```python
from build123d import *

# Parameters (mm, degrees)
SKETCH1_W           = 152.4
SKETCH1_H           = 76.2
BOSS_EXTRUDE1_DEPTH = 25.4
SKETCH2_R           = 6.35
CUT_EXTRUDE1_DEPTH  = 89.9
SKETCH3_R           = 28.575
BOSS_EXTRUDE2_DEPTH = 19.05
SKETCH4_R           = 15.875
CUT_EXTRUDE3_DEPTH  = 97.092936785
FILLET1_R           = 6.35
CHAMFER1_SIZE       = 3.175


with BuildPart() as part:
    # Sketch1 → Boss-Extrude1 (new body)
    with BuildSketch(Plane(origin=(0, 0, 0), x_dir=(1, 0, 0), z_dir=(0, 1, 0))):
        Rectangle(SKETCH1_W, SKETCH1_H)
    extrude(amount=BOSS_EXTRUDE1_DEPTH)

    # Sketch2 → Cut-Extrude1 (cut, through all)
    with BuildSketch(Plane(origin=(0, 25.4, 0), x_dir=(1, 0, 0), z_dir=(0, 1, 0))):
        with Locations(Location((-57.15, 19.05, 0), (0, 0, 270))):
            Circle(SKETCH2_R)
        with Locations(Location((-57.15, -19.05, 0), (0, 0, 90))):
            Circle(SKETCH2_R)
        with Locations(Location((57.15, -19.05, 0), (0, 0, 270))):
            Circle(SKETCH2_R)
        with Locations(Location((57.15, 19.05, 0), (0, 0, 90))):
            Circle(SKETCH2_R)
    extrude(amount=-CUT_EXTRUDE1_DEPTH, mode=Mode.SUBTRACT)

    # Sketch3 → Boss-Extrude2 (add)
    with BuildSketch(Plane(origin=(0, 25.4, 0), x_dir=(1, 0, 0), z_dir=(0, 1, 0))):
        with Locations(Location((0, 0, 0), (0, 0, 90))):
            Circle(SKETCH3_R)
    extrude(amount=BOSS_EXTRUDE2_DEPTH)

    # Sketch4 → Cut-Extrude3 (cut, through all)
    with BuildSketch(Plane(origin=(0, 44.45, 0), x_dir=(1, 0, 0), z_dir=(0, 1, 0))):
        with Locations(Location((0, 0, 0), (0, 0, 270))):
            Circle(SKETCH4_R)
    extrude(amount=-CUT_EXTRUDE3_DEPTH, mode=Mode.SUBTRACT)

    # Fillet1
    fillet1_edges = [part.edges().sort_by_distance(p)[0] for p in [
        (0, 25.4, 28.575),
        (76.2, 12.7, 38.1),
        (-76.2, 12.7, 38.1),
        (-76.2, 12.7, -38.1),
        (76.2, 12.7, -38.1),
    ]]
    fillet(fillet1_edges, radius=FILLET1_R)

    # Chamfer1
    chamfer1_edges = [part.edges().sort_by_distance(p)[0] for p in [
        (76.2, 25.4, 0),
        (0, 25.4, -38.1),
        (-76.2, 25.4, 0),
        (0, 25.4, 38.1),
        (-74.340128061, 25.4, 36.240128061),
        (74.340128061, 25.4, 36.240128061),
        (74.340128061, 25.4, -36.240128061),
        (-74.340128061, 25.4, -36.240128061),
    ]]
    chamfer(chamfer1_edges, length=CHAMFER1_SIZE - 0.0001)  # a hair under: the kernel refuses the full size


solid = part.part
```
Input: part model. Units: mm. Frame: model coordinates. A direction names the side the tool comes from. Round coordinates to 2 decimals unless told otherwise and drop trailing zeros. Write each loop counter-clockwise with the first axis right and the second up, starting at its lowest first coordinate (ties: lowest second). Pieces come first, ordered by that corner, then holes. Notation, with made-up numbers: (21, 32) - (71, 32) arc R20 cw to (71, 38) - close; hole circle Ø10 at (40.5, 37.25). An arc over 180 degrees is marked (long way). Write item = value, one per line.
(1) Material intervals for probe 1 along X at (y, z) = (19, -19); probe 2 along Z at (x, y) = (-57, 5); probe 3 along X at (y, z) = (22.5, -22), sorted ascending.
Geometry check:
probe_1 = -76.2 to -63.5, -50.8 to 50.8, 63.5 to 76.2
probe_2 = -38.1 to -25.4, -12.7 to 12.7, 25.4 to 38.1
probe_3 = -75.93 to -62.77, -51.53 to 51.53, 62.77 to 75.93
(2) Access query for faces 4 (the flat face through (74.635, 23.79, 0.444)), 5 (the flat face through (-17, 25.4, -32)). Directions: +Z, -Z, +X, -X, +Y, -Y. A direction counts if a zero-diameter tool reaches every point of the face in a straight line with its end or side. Return the directions, or none.
Geometry check:
face_4 = +Z, -Z, +X, +Y
face_5 = +Y
(3) Section query C-C on y = 17. Output: boundary loops of the cut face in (x, z) (3 decimals), then the cut area to 3 significant figures.
Geometry check:
outline = (-76.2, -31.75) arc R6.35 ccw to (-69.85, -38.1) - (69.85, -38.1) arc R6.35 ccw to (76.2, -31.75) - (76.2, 31.75) arc R6.35 ccw to (69.85, 38.1) - (-69.85, 38.1) arc R6.35 ccw to (-76.2, 31.75) - close; hole circle Ø12.7 at (-57.15, -19.05); hole circle Ø12.7 at (-57.15, 19.05); hole circle Ø31.75 at (0, 0); hole circle Ø12.7 at (57.15, -19.05); hole circle Ø12.7 at (57.15, 19.05)
area = 10,300 mm^2
(4) Section query B-B on z = 0. Output: boundary loops of the cut face in (x, y) (3 decimals).
Geometry check:
outline = (-76.2, 0) - (-15.875, 0) - (-15.875, 44.45) - (-28.575, 44.45) - (-28.575, 31.75) arc R6.35 cw to (-34.925, 25.4) - (-73.025, 25.4) - (-76.2, 22.225) - close; (15.875, 0) - (76.2, 0) - (76.2, 22.225) - (73.025, 25.4) - (34.925, 25.4) arc R6.35 cw to (28.575, 31.75) - (28.575, 44.45) - (15.875, 44.45) - close
(5) Section query D-D on x = 39. Output: boundary loops of the cut face in (y, z), then the cut area to 3 significant figures.
Geometry check:
outline = (0, -38.1) - (22.23, -38.1) - (25.4, -34.93) - (25.4, 34.93) - (22.23, 38.1) - (0, 38.1) - close
area = 1,930 mm^2
(6) Contact query for flat-ended pins moving along their axis: pin 1 Ø10 at (x, z) = (57.15, -19.05) entering from +Y; pin 2 Ø6 at (y, z) = (31.5, -3.5) entering from -X; pin 3 Ø6 at (x, z) = (-35, -11.5) entering from +Y; pin 4 Ø4 at (y, z) = (33, -4.5) entering from -X. Output: stop coordinate, or through.
Geometry check:
pin_1 = through
pin_2 = -29.29
pin_3 = 25.49
pin_4 = -28.47
(7) Pull-direction query (Z, two-part tool) for faces 1 (the flat face through (-0.978, 23.79, 36.535)), 2 (the cylindrical face through (55.243, 12.878, -25.107)), 3 (the conical face through (73.02, 24.14, -34.85)); classes: +Z half, -Z half, draft (parallel to the pull), parting line (faces both ways), or undercut.
Geometry check:
face_1 = +Z half
face_2 = undercut
face_3 = -Z half
